Drawing for the job (mm, zero at the part's lowest x, y, z). A direction names the side the tool comes from. Round coordinates to 2 decimals unless told otherwise and drop trailing zeros. Loops run counter-clockwise (first coordinate to the right, second up) from the corner with the lowest first, then second, coordinate; pieces in that order, holes last.
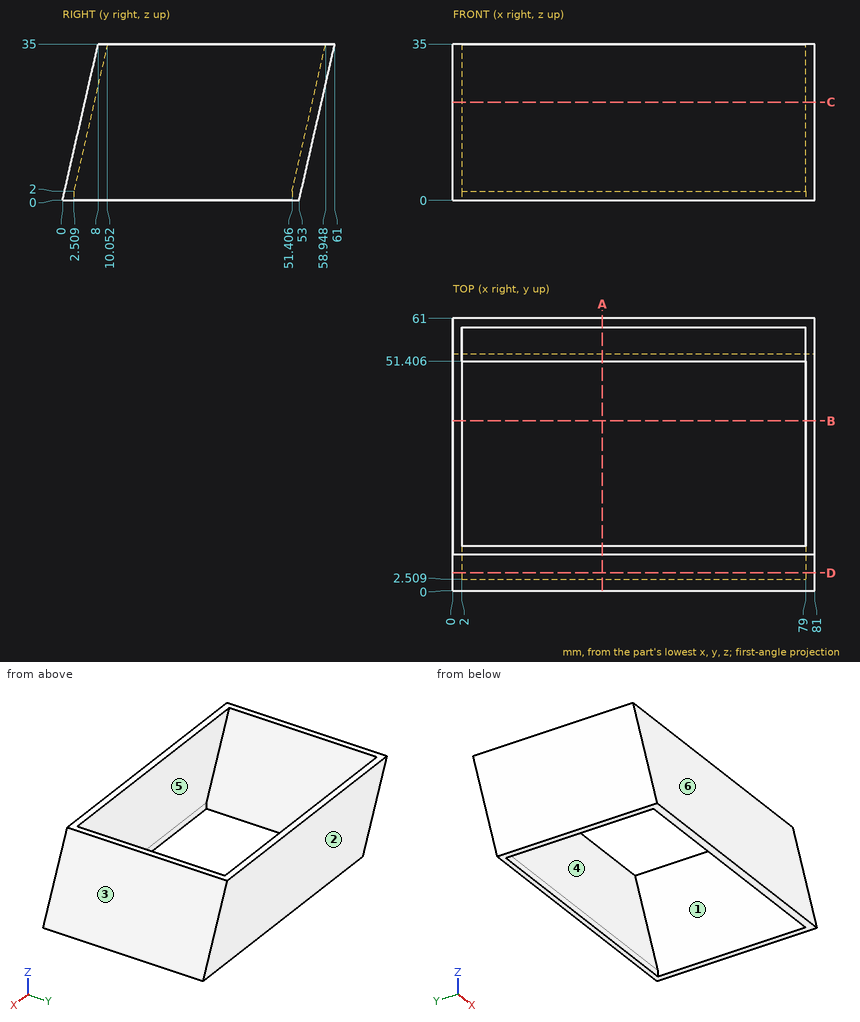
Q1. Pull direction Y, two halves, no side cores. Call the marked faces 1, 2 and 3: pulls with the +Y half, pulls with the -Y half, needs draft (parallel to the pull), parting line crosses it, or undercut.
Q2. Tool access for the marked faces 4, 5 and 6: list every direction of +Z, -Z, +X, -X, +Y, -Y with a clear straight run to the whole face (end or side of a thin tool).
Q3. Slice it at C-C on z = 22. Give the cut face in (x, y).
Q4. Slice it at B-B on y = 38. Give the cut face in (x, z), plus the area to 3 significant figures.
Q5. Flat gauge pins, fed straight in: P1, Ø6, axis at x = 21, z = 18.5, coming from the -Y side; P2, Ø0.6, axis at x = 55, z = 1, coming from the -Y side; P3, Ø8, axis at x = 39, z = 12, coming from the -Y side. Where does each tip first touch, or does it go through?
Q6. Slice it at A-A on x = 33.5. Give the cut face in (y, z) (1 decimal).
Q7. Probe line 1 (X direction, y = 9, z = 3.5); line 2 (Y direction, x = 43, z = 32) (1 decimal); line 3 (Y direction, x = 47.5, z = 3) (1 decimal). List the from-to ranges inside material, lowest first.
Q8. Slice it at D-D on y = 4. Give the cut face in (x, z) (1 decimal), plus the area to 3 significant figures.
Reply:
1. face 1: undercut
1. face 2: pulls with the +Y half
1. face 3: needs draft
2. face 4: +Z
2. face 5: -Z
2. face 6: +Z, +X, -X, -Y
3. outline: (0, 5.03) - (81, 5.03) - (81, 58.03) - (0, 58.03) - close; hole (2, 7.08) - (79, 7.08) - (79, 55.98) - (2, 55.98) - close
4. outline: (0, 0) - (2, 0) - (2, 35) - (0, 35) - close; (79, 0) - (81, 0) - (81, 35) - (79, 35) - close
4. area: 140 mm2
5. P1: stops at y = 3.54
5. P2: stops at y = 0.16
5. P3: stops at y = 1.83
6. outline: (0, 0) - (2.5, 0) - (2.5, 2) - (10.1, 35) - (8, 35) - close; (51.4, 0) - (53, 0) - (61, 35) - (58.9, 35) - (51.4, 2) - close
7. line 1: x = 0 to 2, 79 to 81
7. line 2: y = 7.3 to 9.4, 58.3 to 60.3
7. line 3: y = 0.7 to 2.7, 51.6 to 53.7
8. outline: (0, 0) - (2, 0) - (2, 8.5) - (79, 8.5) - (79, 0) - (81, 0) - (81, 17.5) - (0, 17.5) - close
8. area: 761 mm2
